Autodesk Inventor part; units mm, degrees
ref_plane "YZ Plane" through (0, 0, 0) normal (1, 0, 0) x (0, 1, 0)
ref_plane "XZ Plane" through (0, 0, 0) normal (0, 1, 0) x (-1, 0, 0)
ref_plane "XY Plane" through (0, 0, 0) normal (0, 0, 1) x (1, 0, 0)
sketch "Sketch3" plane through (0, 0, 0) normal (0, 0, 1) x (1, 0, 0)
  line L0 (0, 0) -> (113.5126, 0)
  line L1 (113.5126, 0) -> (113.5126, 6.35)
  line L2 (113.5126, 6.35) -> (3.9624, 6.35)
  line L3 (3.9624, 6.35) -> (3.9624, 17.4625)
  line L4 (3.9624, 17.4625) -> (0, 17.4625)
  line L5 (0, 17.4625) -> (0, 0)
  line L6 (0, 17.4625) -> (0, 18.415) construction
  line L7 (0, 18.415) -> (113.5126, 18.415) construction
  line L8 (113.5126, 18.415) -> (113.5126, 0) construction
  dimension "d163" = 113.5126
  dimension "d164" = 6.35
  dimension "d165" = 109.5502
  dimension "d166" = 11.1125
  dimension "d167" = 0.9525
revolve "Revolution2" add sketch "Sketch3" angle 360 about axis through (0, 18.415, 0) along (1, 0, 0)
fillet "Fillet1" radius 6.35 1 edges at (0, 36.83, 0)
fillet "Fillet2" radius 6.35 1 edges at (113.5126, 36.83, 0)
properties part number "5.5 Sleeve Handle" material "Rubber"
Source: CAD feature listing. Evaluate the final solid. Frame: model axes, mm. A direction names the side the tool comes from. Coordinates: 2 decimals unless noted, no trailing zeros. Loops run counter-clockwise (first coordinate to the right, second up) from the corner with the lowest first, then second, coordinate; pieces in that order, holes last. Notation, with made-up numbers: (88, 59.5) -> (111, 59.5) arc R22 cw to (111, 78.5) -> close; hole circle Ø9 at (57.25, 78.5). An arc over 180 degrees is marked (long way). Answer in a Markdown table with one row per item. Add a question column.
Q1. Pull-direction query (Y, two-part tool) for faces 1 (the face through (3.962, 19, 3)), 2 (the face through (0, 19, 3)), 3 (the face through (57.462, 33.029, 11.205)); classes: pulls with the +Y half, pulls with the -Y half, needs draft (parallel to the pull), parting line crosses it, or undercut.
Q2. Ray query, line 1 along Y through (x, z) = (54, 0); line 2 along Z through (x, y) = (38, 19); line 3 along Z through (x, y) = (66.5, 17). Return the intervals inside material, ascending.
Q3. Section A-A on x = 43. Return the cut outline in (y, z) (3 decimals).
Q4. Reachability of faces 4 (the face through (1.953, 19.367, 0.042)), 5 (the face through (58, 6.9, 3.6)) from +Z, -Z, +X, -X, +Y, -Y: full face, straight path, thin tool, end or side. Return the list, or none.
Q5. Contact query for flat-ended pins moving along their axis: pin 1 Ø3 at (x, y) = (16, 9.5) entering from +Z; pin 2 Ø2 at (x, y) = (81.5, 18.5) entering from +Z (3 decimals); pin 3 Ø3 at (y, z) = (18.415, 0) entering from +X. Output: stop coordinate, or through.
Computed values:
| question | item | result |
|---|---|---|
| 1 | face 1 | undercut |
| 1 | face 2 | needs draft |
| 1 | face 3 | parting line crosses it |
| 2 | line 1 | y = 0 to 6.35, 30.48 to 36.83 |
| 2 | line 2 | z = -18.41 to -12.05, 12.05 to 18.41 |
| 2 | line 3 | z = -18.36 to -11.98, 11.98 to 18.36 |
| 3 | outline | circle Ø36.83 at (18.415, 0); hole circle Ø24.13 at (18.415, 0) |
| 4 | face 4 | +X, -X |
| 4 | face 5 | +X |
| 5 | pin 1 | stops at z = 16.86 |
| 5 | pin 2 | stops at z = 18.415 |
| 5 | pin 3 | stops at x = 3.96 |
